from build123d import *

# Parameters (mm, degrees)
F1_DEPTH = 25
F2_R     = 3
F3_W     = 25
F3_H     = 2
F4_DEPTH = 3
F5_W     = 1.6
F5_H     = 20
F6_DEPTH = 12.5
F7_R     = 3


with BuildPart() as f1:
    # F0 (on Front) → F1 (new body)
    with BuildSketch(Plane.XZ):
        Polygon((2, 5), (0, 5), (0, 0), (5, 0), (5, 1.95942), (2, 1.95942), align=None)
    extrude(amount=F1_DEPTH)

    # F2
    f2_edges = [f1.edges().sort_by_distance(p)[0] for p in [
        (0, -12.5, 0),
    ]]
    fillet(f2_edges, radius=F2_R)

    # F3 (on face) → F4 (join)
    with BuildSketch(Plane(origin=(0, 0, 0), x_dir=(0, -1, 0), z_dir=(-1, 0, 0))):
        with Locations((12.5, 4)):
            Rectangle(F3_W, F3_H)
    extrude(amount=F4_DEPTH)

    # F5 (on face) → F6 (cut, symmetric)
    with BuildSketch(Plane.XY.offset(5)):
        with Locations((-0.8, -12.5)):
            Rectangle(F5_W, F5_H)
    extrude(amount=F6_DEPTH, both=True, mode=Mode.SUBTRACT)

    # F7
    f7_edges = [f1.edges().sort_by_distance(p)[0] for p in [
        (-3, 0, 4),
        (-3, -25, 4),
    ]]
    fillet(f7_edges, radius=F7_R)


solid = f1.part
Verification items for the finished model (mm, model axes). A direction names the side the tool comes from. Give positions to 0.01 mm unless a question says otherwise; leave off trailing zeros. Loops run counter-clockwise (first coordinate to the right, second up) from the corner with the lowest first, then second, coordinate; pieces in that order, holes last.
1. Cross-section at C-C on x = -0.5. Record the cut outline in (y, z).
Derived:
outline: (-24.96, 3) - (-22.5, 3) - (-22.5, 5) - (-24.96, 5) - close; (-2.5, 3) - (-0.04, 3) - (-0.04, 5) - (-2.5, 5) - close
2. Tool access check on faces 1 (the flat face through (5, -12, 1)), 2 (the flat face through (-2, -12, 3)), 3 (the flat face through (0, -13, 4)), 4 (the flat face through (2, -12, 3)). Record the directions out of +Z, -Z, +X, -X, +Y, -Y that give a thin tool (end or side, any length) a straight path to the whole face; none if there is none.
Derived:
face 1: +Z, -Z, +X, +Y, -Y
face 2: -Z, -X, +Y, -Y
face 3: +Z, -Z
face 4: +Z, +X, +Y, -Y
3. Cross-section at B-B on z = 4.1. Record the cut outline in (x, y), and give its area (3 significant figures).
Derived:
outline: (-3, -22) arc R3 ccw to (0, -25) - (2, -25) - (2, 0) - (0, 0) arc R3 ccw to (-3, -3) - close; hole (-1.6, -22.5) - (0, -22.5) - (0, -2.5) - (-1.6, -2.5) - close
area: 89.1 mm2
4. Cross-section at D-D on x = 4. Record the cut outline in (y, z), and give its area (3 significant figures).
Derived:
outline: (-25, 0) - (0, 0) - (0, 1.96) - (-25, 1.96) - close
area: 49.0 mm2
5. Material ranges on probe 1 along X at (y, z) = (-12.75, 3.2); probe 2 along Z at (x, y) = (-0.5, -24); probe 3 along Y at (x, z) = (-0.5, 4.2), recorded low to high.
Derived:
probe 1: x = -3 to -1.6, 0 to 2
probe 2: z = 3 to 5
probe 3: y = -24.96 to -22.5, -2.5 to -0.04
6. Cross-section at A-A on y = -19.5. Record the cut outline in (x, z), and give its area (3 significant figures).
Derived:
outline: (-3, 3) - (-1.6, 3) - (-1.6, 5) - (-3, 5) - close; (0, 3) arc R3 ccw to (3, 0) - (5, 0) - (5, 1.96) - (2, 1.96) - (2, 5) - (0, 5) - close
area: 16.7 mm2
7. Go/stop test with flat-tipped pins: P1, Ø1.5, axis at y = -10.5, z = 3, coming from the +X side; P2, Ø0.8, axis at x = -1, z = 4.5, coming from the -Y side; P3, Ø2.5, axis at x = -1.5, y = -11, coming from the -Z side. Record where each tip stops, or that it passes through.
Derived:
P1: stops at x = 2
P2: stops at y = -24.94
P3: stops at z = 3
